Part model, mm, in its own coordinate system. A direction names the side the tool comes from. Round coordinates to 2 decimals unless told otherwise and drop trailing zeros. Order: outer loops, then holes, each group sorted by start corner. A loop starts at its lowest first (then second) coordinate and runs counter-clockwise, first axis right, second up. Notation, with made-up numbers: (30, -6) - (60, -6) arc R25 cw to (60, 20) - close; hole circle Ø7 at (67.5, -33). An arc over 180 degrees is marked (long way). Answer as a JSON object with one key per item and string values.
Solid Edge part; units mm, degrees
sketch "Sketch1" plane through (0, 0, 0) normal (0, 0, 1) x (1, 0, 0)
  line L0 (-34, -17) -> (34, -17)
  line L1 (34, -17) -> (34, 17)
  line L2 (34, 17) -> (-34, 17)
  line L3 (-34, 17) -> (-34, -17)
  circle A0 centre (-29, -13) radius 1.7
  circle A1 centre (-29, 13) radius 1.7
  circle A2 centre (29, -13) radius 1.7
  circle A3 centre (29, 13) radius 1.7
extrude "Protrusion1" add sketch "Sketch1" along normal blind 3
sketch "Sketch2" plane through (0, 0, 3) normal (0, 0, 1) x (1, 0, 0)
  line L0 (-26, -11) -> (26, -11)
  line L1 (26, -11) -> (26, 11)
  line L2 (26, 11) -> (-26, 11)
  line L3 (-26, 11) -> (-26, -11)
  line L4 (-24.5, -9.5) -> (24.5, -9.5)
  line L5 (24.5, -9.5) -> (24.5, 9.5)
  line L6 (24.5, 9.5) -> (-24.5, 9.5)
  line L7 (-24.5, 9.5) -> (-24.5, -9.5)
extrude "ExtrudedProtrusion_2" add sketch "Sketch2" along normal blind 6
sketch "Sketch3" plane through (0, 0, 3) normal (0, 0, 1) x (1, 0, 0)
  circle A0 centre (0, -13) radius 3.5
  circle A1 centre (0, -13) radius 1.7
  circle A2 centre (0, 13) radius 3.5
  circle A3 centre (0, 13) radius 1.7
extrude "ExtrudedProtrusion_3" add sketch "Sketch3" along normal blind 15.9
sketch "Sketch4" plane through (0, 0, 16.2) normal (0, 0, 1) x (1, 0, 0)
  line L0 (3.3486, -13) -> (1.6743, -10.1)
  line L1 (1.6743, -10.1) -> (-1.6743, -10.1)
  line L2 (-1.6743, -10.1) -> (-3.3486, -13)
  line L3 (-3.3486, -13) -> (-1.6743, -15.9)
  line L4 (-1.6743, -15.9) -> (1.6743, -15.9)
  line L5 (1.6743, -15.9) -> (3.3486, -13)
  line L6 (3.3486, 13) -> (1.6743, 15.9)
  line L7 (1.6743, 15.9) -> (-1.6743, 15.9)
  line L8 (-1.6743, 15.9) -> (-3.3486, 13)
  line L9 (-3.3486, 13) -> (-1.6743, 10.1)
  line L10 (-1.6743, 10.1) -> (1.6743, 10.1)
  line L11 (1.6743, 10.1) -> (3.3486, 13)
extrude "ExtrudedCutout_1" cut sketch "Sketch4" along normal blind 2.7
Item 1: Cut at C-C (z = 14). Write the cut outline in (x, y).
Taken from the geometry:
{"outline": "circle Ø7 at (0, -13); circle Ø7 at (0, 13); hole circle Ø3.4 at (0, -13); hole circle Ø3.4 at (0, 13)"}
Item 2: Cut at A-A (x = 29). Write the cut outline in (y, z).
Taken from the geometry:
{"outline": "(-17, 0) - (-14.7, 0) - (-14.7, 3) - (-17, 3) - close; (-11.3, 0) - (11.3, 0) - (11.3, 3) - (-11.3, 3) - close; (14.7, 0) - (17, 0) - (17, 3) - (14.7, 3) - close"}
Item 3: Cut at D-D (y = 7). Write the cut outline in (x, z), plus the area to 3 significant figures.
Taken from the geometry:
{"outline": "(-34, 0) - (34, 0) - (34, 3) - (26, 3) - (26, 9) - (24.5, 9) - (24.5, 3) - (-24.5, 3) - (-24.5, 9) - (-26, 9) - (-26, 3) - (-34, 3) - close", "area": "222 mm2"}
Item 4: Tool access for faces 1 (the cylindrical face through (-0.221, 11.314, 9.508)), 2 (the flat face through (34, 0, 1)), 3 (the flat face through (-26, 0, 6)): list every direction of +Z, -Z, +X, -X, +Y, -Y with a clear straight run to the whole face (end or side of a thin tool).
Taken from the geometry:
{"face 1": "+Z", "face 2": "+Z, -Z, +X, +Y, -Y", "face 3": "+Z, -X, +Y, -Y"}
Item 5: Cut at B-B (z = 5). Write the cut outline in (x, y), plus the area to 3 significant figures.
Taken from the geometry:
{"outline": "(-26, -11) - (-2.87, -11) arc R3.5 ccw (long way) to (2.87, -11) - (26, -11) - (26, 11) - (2.87, 11) arc R3.5 ccw (long way) to (-2.87, 11) - (-26, 11) - close; hole (-24.5, -9.5) - (24.5, -9.5) - (24.5, 9.5) - (-24.5, 9.5) - close; hole circle Ø3.4 at (0, -13); hole circle Ø3.4 at (0, 13)", "area": "260 mm2"}
Item 6: Two-plate mould, pull along X, no slides. Class faces 4 (the flat face through (-34, 0, 1)), 5 (the flat face through (24.5, 0, 6)), 6 (the flat face through (25, 0, 9)), 7 (the flat face through (2.5, -14.47, 17.53)): pulls with the +X half, pulls with the -X half, needs draft (parallel to the pull), parting line crosses it, or undercut.
Taken from the geometry:
{"face 4": "pulls with the -X half", "face 5": "undercut", "face 6": "needs draft", "face 7": "undercut"}
Item 7: Drop flat-ended pins along their axis: P1, Ø0.8, axis at x = -0.5, z = 18, coming from the -Y side; P2, Ø1, axis at x = -3.5, y = -4, coming from the -Z side; P3, Ø1, axis at x = -2, z = 6.5, coming from the +Y side; P4, Ø3, axis at x = 0, z = 5.5, coming from the +Y side. Give the stop position or say it passes through.
Taken from the geometry:
{"P1": "y = -16.5", "P2": "z = 0", "P3": "y = 16.16", "P4": "y = 16.5"}
Item 8: Probe L1, parallel to Y at x = 0, z = 13; L2, parallel to Y at x = 29, z = 0.8; L3, parallel to X at y = -13, z = 5.5. List the from-to ranges inside material, lowest first. Write a range as from..to.
Taken from the geometry:
{"L1": "-16.5..-14.7, -11.3..-9.5, 9.5..11.3, 14.7..16.5", "L2": "-17..-14.7, -11.3..11.3, 14.7..17", "L3": "-3.5..-1.7, 1.7..3.5"}
